Part model, mm, in its own coordinate system. A direction names the side the tool comes from. Give positions to 0.01 mm unless a question says otherwise; leave off trailing zeros. Write each loop counter-clockwise with the first axis right and the second up, starting at its lowest first coordinate (ties: lowest second). Pieces come first, ordered by that corner, then holes.
```python
from build123d import *

# Parameters (mm, degrees)
BOSS_EXTRUDE1_DEPTH             = 19.05
F_7_32_0_21875_DIAMETER_HOLE3_D = 5.55625


with BuildPart() as part:
    # Sketch1 → Boss-Extrude1 (new body)
    with BuildSketch(Plane(origin=(0, 0, 0), x_dir=(0, 0, -1), z_dir=(1, 0, 0))):
        Polygon((19.05, 0), (177.8635, 0), (177.8635, 114.3), (19.05, 114.3), (19.05, 101.6), (0, 101.6), (0, 88.9), (19.05, 88.9), (19.05, 76.2), (0, 76.2), (0, 63.5), (19.05, 63.5), (19.05, 50.8), (0, 50.8), (0, 38.1), (19.05, 38.1), (19.05, 25.4), (0, 25.4), (0, 12.7), (19.05, 12.7), align=None)
    extrude(amount=BOSS_EXTRUDE1_DEPTH)

    # 7/32 (0.21875) Diameter Hole3 (through all)
    with Locations(Plane(origin=(19.05, 0, 0), x_dir=(0, 0, -1), z_dir=(1, 0, 0))):
        with Locations((42.7101, 19.05), (153.9875, 55.499), (98.3488, 55.499), (42.7101, 55.499), (42.7101, 95.25)):
            Hole(F_7_32_0_21875_DIAMETER_HOLE3_D / 2)


solid = part.part
```
1) Wall check: L1, parallel to Y at x = 1.25, z = -15; L2, parallel to Y at x = 12.5, z = -45; L3, parallel to Z at x = 16, y = 19. Give the ranges that are in metal, low to high.
Answers follow:
L1: y = 12.7 to 25.4, 38.1 to 50.8, 63.5 to 76.2, 88.9 to 101.6
L2: y = 0 to 17.48, 20.62 to 53.93, 57.07 to 93.68, 96.82 to 114.3
L3: z = -177.86 to -45.49, -39.93 to 0
2) Saw through at B-B, the plane x = 8.75. Write the cut outline in (y, z).
Answers follow:
outline: (0, -177.86) - (114.3, -177.86) - (114.3, -19.05) - (101.6, -19.05) - (101.6, 0) - (88.9, 0) - (88.9, -19.05) - (76.2, -19.05) - (76.2, 0) - (63.5, 0) - (63.5, -19.05) - (50.8, -19.05) - (50.8, 0) - (38.1, 0) - (38.1, -19.05) - (25.4, -19.05) - (25.4, 0) - (12.7, 0) - (12.7, -19.05) - (0, -19.05) - close; hole circle Ø5.56 at (19.05, -42.71); hole circle Ø5.56 at (55.5, -153.99); hole circle Ø5.56 at (55.5, -98.35); hole circle Ø5.56 at (55.5, -42.71); hole circle Ø5.56 at (95.25, -42.71)
3) Saw through at A-A, the plane y = 19.05. Write the cut outline in (x, z), then the cut area to 3 significant figures.
Answers follow:
outline: (0, -177.86) - (19.05, -177.86) - (19.05, -45.49) - (0, -45.49) - close; (0, -39.93) - (19.05, -39.93) - (19.05, 0) - (0, 0) - close
area: 3,280 mm2
4) 3-axis set-ups, long thin cutter, end or side, ignore diameter. For faces 4 (the face through (9, 101.6, -10)), 5 (the face through (9, 114.3, -100)), 6 (the face through (9, 45, 0)), 7 (the face through (9, 32, -19.05)), 8 (the face through (9, 6, -19.05)): which of +Z, -Z, +X, -X, +Y, -Y reach the whole face in a straight line?
Answers follow:
face 4: +Z, +X, -X, +Y
face 5: +Z, -Z, +X, -X, +Y
face 6: +Z, +X, -X, +Y, -Y
face 7: +Z, +X, -X
face 8: +Z, +X, -X, -Y
5) Saw through at C-C, the plane y = 33. Write the cut outline in (x, z).
Answers follow:
outline: (0, -177.86) - (19.05, -177.86) - (19.05, -19.05) - (0, -19.05) - close
6) Pin check, flat tip, straight feed: pin 1 Ø6.5 at (x, y) = (5, 5.5) entering from +Z. Stop position of the tip, or through.
Answers follow:
pin 1: stops at z = -19.05
7) Two-plate mould, pull along Z, no slides. Class faces 1 (the face through (9, 25.4, -10)), 2 (the face through (9.392, 55.621, -156.763)), 3 (the face through (9, 56, -177.864)): +Z half, -Z half, draft (parallel to the pull), parting line (faces both ways), or undercut.
Answers follow:
face 1: draft
face 2: undercut
face 3: -Z half
